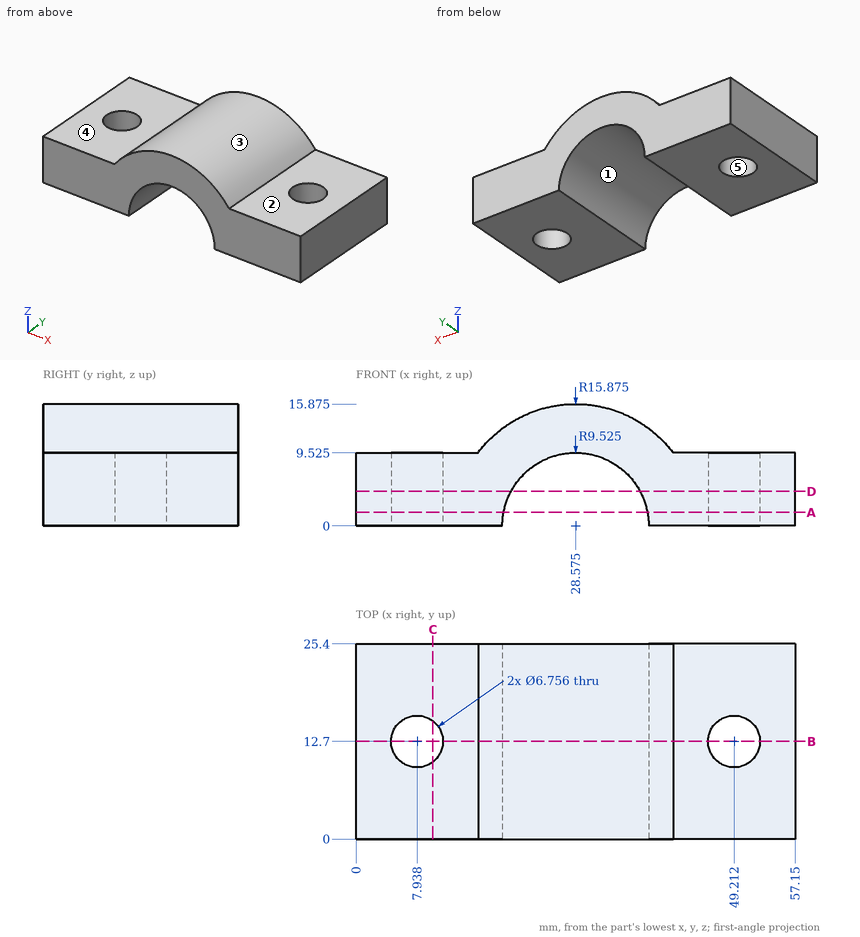
Can you work these out from the drawing? Everything is in mm from the part's minimum corner. A direction names the side the tool comes from. Round coordinates to 2 decimals unless told otherwise and drop trailing zeros. Loops run counter-clockwise (first coordinate to the right, second up) from the corner with the lowest first, then second, coordinate; pieces in that order, holes last. Notation, with made-up numbers: (-33, 43.5) -> (-1, 43.5) arc R31 ccw to (-1, 76.5) -> close; hole circle Ø9 at (45.5, -5.75). An arc over 180 degrees is marked (long way). Use CSV: the item, a comma, the result in double quotes.
(1) If we mould it in two halves opening along X, with no side actions, what happens to the marked faces 1, 2 and 3? For each: +X half, -X half, draft (parallel to the pull), parting line (faces both ways), or undercut.
Return value:
face 1,"undercut"
face 2,"draft"
face 3,"parting line"
(2) Suppose I cut it at A-A on z = 1.75. Write out the boundary of the cut face in (x, y), plus the area to 3 significant figures.
Return value:
outline,"(0, 0) -> (19.21, 0) -> (19.21, 25.4) -> (0, 25.4) -> close; (37.94, 0) -> (57.15, 0) -> (57.15, 25.4) -> (37.94, 25.4) -> close; hole circle Ø6.76 at (7.94, 12.7); hole circle Ø6.76 at (49.21, 12.7)"
area,"904 mm²"
(3) For the marked faces 4 and 5, which set-ups out of +Z, -Z, +X, -X, +Y, -Y let a thin tool reach every point of the face, with its end or its side?
Return value:
face 4,"+Z, -X, +Y, -Y"
face 5,"+Z, -Z"
(4) Suppose I cut it at D-D on z = 4.5. Write out the boundary of the cut face in (x, y).
Return value:
outline,"(0, 0) -> (20.18, 0) -> (20.18, 25.4) -> (0, 25.4) -> close; (36.97, 0) -> (57.15, 0) -> (57.15, 25.4) -> (36.97, 25.4) -> close; hole circle Ø6.76 at (7.94, 12.7); hole circle Ø6.76 at (49.21, 12.7)"
(5) If I drill on probe 1 along Z at (x, y) = (54.5, 1.75) (1 decimal); probe 2 along Z at (x, y) = (16, 12); probe 3 along Y at (x, z) = (51.5, 2.75) (1 decimal), over which ranges is the centre line in solid material (lowest first)? Write a range as [from, to].
Return value:
probe 1,"z = [0, 9.5]"
probe 2,"z = [0, 9.69]"
probe 3,"y = [0, 10.2], [15.2, 25.4]"
(6) Suppose I cut it at C-C on x = 10. Write out the boundary of the cut face in (y, z) (1 decimal).
Return value:
outline,"(0, 0) -> (10, 0) -> (10, 9.5) -> (0, 9.5) -> close; (15.4, 0) -> (25.4, 0) -> (25.4, 9.5) -> (15.4, 9.5) -> close"
(7) Suppose I cut it at B-B on y = 12.7. Give the number of separate pieces and of enclosed holes in the cut face, plus the area to 3 significant figures.
Return value:
separate pieces,"3"
enclosed holes,"0"
area,"386 mm²"
(8) Will these pins go through, and if not, where does the flat tip stop? pin 1 Ø1 at (y, z) = (11.5, 11.5) entering from +X; pin 2 Ø1 at (x, y) = (49.5, 8.5) entering from +Z (1 decimal).
Return value:
pin 1,"stops at x = 40.02"
pin 2,"stops at z = 9.5"
